Check sheet for the modelled part. Datum: model origin and axes. Units: mm. Face numbers are marked on the shaded views. A direction names the side the tool comes from. Round coordinates to 2 decimals unless told otherwise and drop trailing zeros. Write each loop counter-clockwise with the first axis right and the second up, starting at its lowest first coordinate (ties: lowest second). Pieces come first, ordered by that corner, then holes. Notation, with made-up numbers: M 24,89 L 78,89 A12 ccw 78,95 Z; hole C -5.5,74 d1. An arc over 180 degrees is marked long. Put each result on its own line as item: value.
```python
from build123d import *

# Parameters (mm, degrees)
SKETCH1_W           = 46
SKETCH1_H           = 28.15
SKETCH1_R           = 1.125
BOSS_EXTRUDE1_DEPTH = 1.5
BOSS_EXTRUDE2_DEPTH = 6.5


with BuildPart() as part:
    # Sketch1 → Boss-Extrude1 (new body)
    with BuildSketch(Plane(origin=(0, 0, 0), x_dir=(1, 0, 0), z_dir=(0, 1, 0))):
        Rectangle(SKETCH1_W, SKETCH1_H)
        with Locations(Location((20.32, -11.43, 0), (0, 0, 270))):
            Circle(SKETCH1_R, mode=Mode.SUBTRACT)
        with Locations(Location((-20.32, -11.43, 0), (0, 0, 90))):
            Circle(SKETCH1_R, mode=Mode.SUBTRACT)
    extrude(amount=BOSS_EXTRUDE1_DEPTH)

    # Sketch2 → Boss-Extrude2 (add)
    with BuildSketch(Plane(origin=(0, 1.5, 0), x_dir=(1, 0, 0), z_dir=(0, 1, 0))):
        with BuildLine():
            Line((-18.07, -11.43), (-18.07, -14.075))
            Line((-18.07, -14.075), (18.07, -14.075))
            Line((18.07, -14.075), (18.07, -11.43))
            ThreePointArc((18.07, -11.43), (18.729009742, -9.839009742), (20.32, -9.18))
            Line((20.32, -9.18), (23, -9.18))
            Line((23, -9.18), (23, 14.075))
            Line((23, 14.075), (-23, 14.075))
            Line((-23, 14.075), (-23, -9.18))
            Line((-23, -9.18), (-20.32, -9.18))
            ThreePointArc((-20.32, -9.18), (-18.729009742, -9.839009742), (-18.07, -11.43))
        make_face()
    extrude(amount=BOSS_EXTRUDE2_DEPTH)


solid = part.part
```
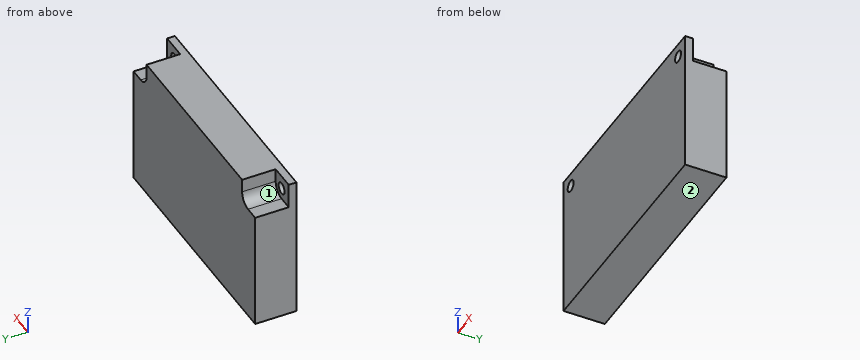
1. Depth check by flat-ended pin: pin 1 Ø2 at (y, z) = (4.5, 12.5) entering from -X; pin 2 Ø1.3 at (y, z) = (5, 12.5) entering from +X; pin 3 Ø2 at (x, y) = (-21.5, 6) entering from +Z. Enter the tip coordinate at first touch or a pass-through.
Computed values:
pin 1: stops at x = -18.07
pin 2: stops at x = 18.07
pin 3: stops at z = 9.18
2. Access from +Z, -Z, +X, -X, +Y, -Y to the whole of each face (thin tool, end or side, straight path). Record for the marked faces 1 and 2.
Computed values:
face 1: +Z, -X, +Y
face 2: -Z, +X, -X, +Y, -Y
3. Cross-section at A-A (y = 6.25). Enter the section's corners in (x, z) (3 decimals).
Computed values:
outline: M -23,-14.075 L 23,-14.075 L 23,9.18 L 20.32,9.18 A2.25 cw 18.07,11.43 L 18.07,14.075 L -18.07,14.075 L -18.07,11.43 A2.25 cw -20.32,9.18 L -23,9.18 Z
4. Scan lines: probe 1 along X at (y, z) = (0.5, 11.43) (3 decimals); probe 2 along Z at (x, y) = (-20.32, 1.1) (3 decimals); probe 3 along Z at (x, y) = (20.5, 5.75) (3 decimals). Record each from-to range of solid material in increasing order.
Computed values:
probe 1: x = -23 to -21.445, -19.195 to 19.195, 21.445 to 23
probe 2: z = -14.075 to 10.305, 12.555 to 14.075
probe 3: z = -14.075 to 9.18
